Design review of the part built by this model. Coordinates are the model's own, in mm. Give positions to 0.01 mm unless a question says otherwise; leave off trailing zeros. Loops run counter-clockwise (first coordinate to the right, second up) from the corner with the lowest first, then second, coordinate; pieces in that order, holes last. Notation, with made-up numbers: (8.5, 3.25) - (39.5, 3.25) arc R23 ccw to (39.5, 24.25) - close; hole circle Ø1 at (5, 41). An arc over 180 degrees is marked (long way). Write each question's results on one line, items separated by ' | '.
from build123d import *

# Parameters (mm, degrees)
SKETCH1_W           = 508
SKETCH1_H           = 304.8
SKETCH1_W_2         = 46.181818182
SKETCH1_H_2         = 6.35
SKETCH1_W_3         = 46.181818181
SKETCH1_W_4         = 3.175
SKETCH1_H_3         = 43.542857143
SKETCH1_H_4         = 43.542857142
BOSS_EXTRUDE1_DEPTH = 3.175
SKETCH2_R           = 1.5
CUT_EXTRUDE1_DEPTH  = 3.175


with BuildPart() as part:
    # Sketch1 → Boss-Extrude1 (new body)
    with BuildSketch(Plane.XY):
        with Locations((254, 152.4)):
            Rectangle(SKETCH1_W, SKETCH1_H)
        with Locations((23.090909091, -3.175)):
            Rectangle(SKETCH1_W_2, SKETCH1_H_2)
        with Locations((115.454545455, -3.175)):
            Rectangle(SKETCH1_W_3, SKETCH1_H_2)
        with Locations((207.818181818, -3.175)):
            Rectangle(SKETCH1_W_2, SKETCH1_H_2)
        with Locations((300.181818182, -3.175)):
            Rectangle(SKETCH1_W_2, SKETCH1_H_2)
        with Locations((392.545454545, -3.175)):
            Rectangle(SKETCH1_W_3, SKETCH1_H_2)
        with Locations((484.909090909, -3.175)):
            Rectangle(SKETCH1_W_2, SKETCH1_H_2)
        with Locations((509.5875, 65.314285715)):
            Rectangle(SKETCH1_W_4, SKETCH1_H_3)
        with Locations((509.5875, 152.4)):
            Rectangle(SKETCH1_W_4, SKETCH1_H_4)
        with Locations((509.5875, 239.485714286)):
            Rectangle(SKETCH1_W_4, SKETCH1_H_3)
        with Locations((-1.5875, 239.485714286)):
            Rectangle(SKETCH1_W_4, SKETCH1_H_3)
        with Locations((-1.5875, 152.4)):
            Rectangle(SKETCH1_W_4, SKETCH1_H_4)
        with Locations((-1.5875, 65.314285715)):
            Rectangle(SKETCH1_W_4, SKETCH1_H_3)
    extrude(amount=BOSS_EXTRUDE1_DEPTH)

    # Sketch2 → Cut-Extrude1 (cut)
    with BuildSketch(Plane.XY.offset(3.175)):
        with Locations((15.875, 274.8)):
            Circle(SKETCH2_R)
        with Locations((15.875, 259.05)):
            Circle(SKETCH2_R)
        with Locations((492.125, 259.05)):
            Circle(SKETCH2_R)
        with Locations((492.125, 274.8)):
            Circle(SKETCH2_R)
    extrude(amount=-CUT_EXTRUDE1_DEPTH, mode=Mode.SUBTRACT)


solid = part.part
(1) Take a section at A-A on z = 2.15. Count the separate pieces of the cut face and the enclosed holes in it, plus the area to 3 significant figures.
Answers below:
separate pieces: 1 | enclosed holes: 4 | area: 157,000 mm2
(2) Insertion check: P1, Ø1.6, axis at x = -1.5, z = 1, coming from the +Y side; P2, Ø1, axis at x = 261.5, z = 2, coming from the -Y side; P3, Ø1, axis at y = 193, z = 2, coming from the -X side. Each pin has a flat end and moves straight along its axis. Give the tip position at first contact, or say it passes through.
Answers below:
P1: y = 261.26 | P2: y = 0 | P3: x = 0
(3) Wall thickness on line 1 along X through (y, z) = (274.8, 1.35) (3 decimals); line 2 along X through (y, z) = (259.05, 1.25) (3 decimals); line 3 along X through (y, z) = (189.5, 1.9): over which ranges is each line inside the solid? List them lowest first. Write a range as from..to.
Answers below:
line 1: 0..14.375, 17.375..490.625, 493.625..508 | line 2: -3.175..14.375, 17.375..490.625, 493.625..511.175 | line 3: 0..508
(4) Take a section at B-B on x = 354. Give the boundary of the cut face in (y, z) (3 decimals), plus the area to 3 significant figures.
Answers below:
outline: (0, 0) - (304.8, 0) - (304.8, 3.175) - (0, 3.175) - close | area: 968 mm2
